The listing builds one solid part. Answer for the finished solid, in the listing's coordinates (mm). Coordinates: 2 decimals unless noted, no trailing zeros. Loops run counter-clockwise (first coordinate to the right, second up) from the corner with the lowest first, then second, coordinate; pieces in that order, holes last. Notation, with made-up numbers: (53, 43.5) - (89, 43.5) arc R28 ccw to (89, 73.5) - close; hole circle Ø7 at (10, -16.5). An arc over 180 degrees is marked (long way). Put each result on its own line as item: value.
```python
from build123d import *

# Parameters (mm, degrees)
SKETCH3_R           = 2.5
BOSS_EXTRUDE1_DEPTH = 5
BOSS_EXTRUDE2_START = -10
SKETCH4_R           = 2.5
SKETCH4_R_2         = 0.5
BOSS_EXTRUDE2_DEPTH = 10
SKETCH5_R           = 2.5
SKETCH5_R_2         = 0.5
BOSS_EXTRUDE3_DEPTH = 8


with BuildPart() as part:
    # Sketch3 → Boss-Extrude1 (new body)
    with BuildSketch(Plane.XY):
        with BuildLine():
            Line((-11.048388083, -10.905646279), (-3.448601602, 2.026609728))
            ThreePointArc((-3.448601602, 2.026609728), (-2.00903777, 3.458867913), (-0.051681177, 3.999666118))
            Line((-0.051681177, 3.999666118), (96.922478234, 5.252705394))
            ThreePointArc((96.922478234, 5.252705394), (102.990943647, -0.417257421), (97.580968918, -6.718600471))
            Line((97.580968918, -6.718600471), (-7.212473869, -16.913460466))
            ThreePointArc((-7.212473869, -16.913460466), (-10.971185359, -15.084852023), (-11.048388083, -10.905646279))
        make_face()
        with Locations((-7.599786481, -12.932256007)):
            Circle(SKETCH3_R, mode=Mode.SUBTRACT)
        Circle(SKETCH3_R, mode=Mode.SUBTRACT)
    extrude(amount=BOSS_EXTRUDE1_DEPTH)

    # Sketch4 → Boss-Extrude2 (add)
    with BuildSketch(Plane.XY.offset(5).offset(BOSS_EXTRUDE2_START)):
        Circle(SKETCH4_R)
        Circle(SKETCH4_R_2, mode=Mode.SUBTRACT)
    extrude(amount=BOSS_EXTRUDE2_DEPTH)

    # Sketch5 → Boss-Extrude3 (add)
    with BuildSketch(Plane(origin=(0, 0, 0), x_dir=(-1, 0, 0), z_dir=(0, 0, -1))):
        with Locations((7.599786481, -12.932256007)):
            Circle(SKETCH5_R)
        with Locations((7.599786481, -12.932256007)):
            Circle(SKETCH5_R_2, mode=Mode.SUBTRACT)
    extrude(amount=-BOSS_EXTRUDE3_DEPTH)


solid = part.part
```
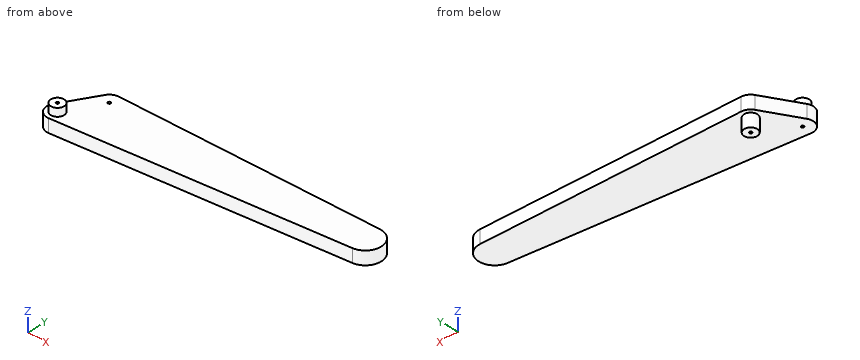
1) Each of these flat-tipped pins is pushed along its axis until it touches: pin 1 (5 mm diameter, centred on y = -7.5, z = 3.5, fed in from +X); pin 2 (6 mm diameter, centred on x = 86.5, y = 2.5, fed in from -Z); pin 3 (4 mm diameter, centred on x = 54.5, z = 6.5, fed in from +Y). Where does it stop, or does it pass through?
Found:
pin 1: stops at x = 101.23
pin 2: stops at z = 0
pin 3: stops at y = 4.72
2) The part is cut by section B-B (x = 57.5). Give the vertices of the cut face in (y, z), and give its area (3 significant figures).
Found:
outline: (-10.62, 0) - (4.74, 0) - (4.74, 5) - (-10.62, 5) - close
area: 76.8 mm^2
3) The part is cut by section A-A (z = 1.75). Give the vertices of the cut face in (x, y).
Found:
outline: (-11.05, -10.91) arc R4 ccw to (-7.21, -16.91) - (97.58, -6.72) arc R6 ccw to (96.92, 5.25) - (-0.05, 4) arc R4 ccw to (-3.45, 2.03) - close; hole circle Ø1 at (-7.6, -12.93); hole circle Ø1 at (0, 0)
4) The part is cut by section C-C (x = 25.5). Give the vertices of the cut face in (y, z).
Found:
outline: (-13.73, 0) - (4.33, 0) - (4.33, 5) - (-13.73, 5) - close
5) Straight lines are drawn through the part: L1, parallel to Y at x = 0, z = -2.5; L2, parallel to Z at x = 49, y = -10.75; L3, parallel to Y at x = 0, z = 2.5. For each, find the intervals that lie inside material, in ascending order. Write a range as [from, to].
Found:
L1: y = [-2.5, -0.5], [0.5, 2.5]
L2: z = [0, 5]
L3: y = [-16.21, -0.5], [0.5, 4]
